```python
from build123d import *

# Parameters (mm, degrees)
SKETCH_1_R          = 4
EXTRUDE_1_DEPTH     = 30
SKETCH_2_R          = 1.7
CUT_EXTRUDE_1_DEPTH = 20


with BuildPart() as part:
    # 草图1 → 凸台-拉伸1 (new body)
    with BuildSketch(Plane.XY):
        Polygon((-17, -7), (-8, -7), (-4, -11), (4, -11), (8, -7), (17, -7), (17, 11), (-17, 11), align=None)
        Circle(SKETCH_1_R, mode=Mode.SUBTRACT)
    extrude(amount=EXTRUDE_1_DEPTH)

    # 草图2 → 切除-拉伸1 (cut)
    with BuildSketch(Plane.XZ.offset(7)):
        with Locations(Location((-12, 24, 0), (0, 0, 270))):
            Circle(SKETCH_2_R)
        with Locations(Location((-12, 6, 0), (0, 0, 270))):
            Circle(SKETCH_2_R)
        with Locations(Location((12, 24, 0), (0, 0, 270))):
            Circle(SKETCH_2_R)
        with Locations(Location((12, 6, 0), (0, 0, 270))):
            Circle(SKETCH_2_R)
    extrude(amount=-CUT_EXTRUDE_1_DEPTH, mode=Mode.SUBTRACT)


solid = part.part
```
Source: CAD feature listing. Evaluate the final solid. Frame: model axes, mm. A direction names the side the tool comes from. Coordinates: 2 decimals unless noted, no trailing zeros. Loops run counter-clockwise (first coordinate to the right, second up) from the corner with the lowest first, then second, coordinate; pieces in that order, holes last. Notation, with made-up numbers: M -2,20 L 22,20 A7 cw 22,25 Z; hole C 29,83 d2. An arc over 180 degrees is marked long. Use a Markdown table: item, result. Add a question column.
Q1. First-contact query: pin 1 (6 mm diameter, centred on x = -6, z = 20.5, fed in from -Y); pin 2 (7 mm diameter, centred on x = -13, z = 17.5, fed in from -Y); pin 3 (2 mm diameter, centred on x = -12, z = 24, fed in from -Y); pin 4 (4 mm diameter, centred on x = -9.5, z = 26, fed in from -Y). Flat tips, straight axial feed; report the tip coordinate or a pass-through.
Q2. Section query B-B, the plane y = 0. Return loops of the section in (x, z), and give its area (3 significant figures).
Q3. Section query A-A, the plane z = 24. Return loops of the section in (x, y).
Q4. Material intervals for L1, parallel to X at y = 5, z = 6; L2, parallel to Z at x = 12.5, y = -2; L3, parallel to X at y = -3, z = 6, sorted ascending.
Q5. Section query D-D, the plane z = 13.5. Return loops of the section in (x, y), and give its area (3 significant figures).
Q6. Draft query along Z for faces 4 (the cylindrical face through (11.35, 1.87, 22.43)), 5 (the flat face through (0, 5, 30)), 6 (the flat face through (-6, -9, 15)), 7 (the flat face through (0, 5, 0)). Return one class per face: pulls with the +Z half, pulls with the -Z half, needs draft (parallel to the pull), parting line crosses it, or undercut.
Q7. Section query C-C, the plane x = -12. Return loops of the section in (y, z), and give its area (3 significant figures).
Q8. Access query for faces 1 (the flat face through (-13, -7, 15)), 2 (the flat face through (12, -7, 15)), 3 (the flat face through (0, -11, 15)). Directions: +Z, -Z, +X, -X, +Y, -Y. A direction counts if a zero-diameter tool reaches every point of the face in a straight line with its end or side. Return the directions, or none.
Result:
| question | item | result |
|---|---|---|
| 1 | pin 1 | stops at y = -11 |
| 1 | pin 2 | stops at y = -7 |
| 1 | pin 3 | passes through |
| 1 | pin 4 | stops at y = -7.5 |
| 2 | outline | M -17,0 L -4,0 L -4,30 L -17,30 Z; M 4,0 L 17,0 L 17,30 L 4,30 Z; hole C -12,6 d3.4; hole C -12,24 d3.4; hole C 12,6 d3.4; hole C 12,24 d3.4 |
| 2 | area | 744 mm2 |
| 3 | outline | M -17,-7 L -13.7,-7 L -13.7,11 L -17,11 Z; M -10.3,-7 L -8,-7 L -4,-11 L 4,-11 L 8,-7 L 10.3,-7 L 10.3,11 L -10.3,11 Z; M 13.7,-7 L 17,-7 L 17,11 L 13.7,11 Z; hole C 0,0 d8 |
| 4 | L1 | x = -17 to -13.7, -10.3 to 10.3, 13.7 to 17 |
| 4 | L2 | z = 0 to 4.38, 7.62 to 22.38, 25.62 to 30 |
| 4 | L3 | x = -17 to -13.7, -10.3 to -2.65, 2.65 to 10.3, 13.7 to 17 |
| 5 | outline | M -17,-7 L -8,-7 L -4,-11 L 4,-11 L 8,-7 L 17,-7 L 17,11 L -17,11 Z; hole C 0,0 d8 |
| 5 | area | 610 mm2 |
| 6 | face 4 | undercut |
| 6 | face 5 | pulls with the +Z half |
| 6 | face 6 | needs draft |
| 6 | face 7 | pulls with the -Z half |
| 7 | outline | M -7,0 L 11,0 L 11,4.3 L -7,4.3 Z; M -7,7.7 L 11,7.7 L 11,22.3 L -7,22.3 Z; M -7,25.7 L 11,25.7 L 11,30 L -7,30 Z |
| 7 | area | 418 mm2 |
| 8 | face 1 | +Z, -Z, -X, -Y |
| 8 | face 2 | +Z, -Z, +X, -Y |
| 8 | face 3 | +Z, -Z, +X, -X, -Y |
